```python
from build123d import *

# Parameters (mm, degrees)
SKETCH1_R           = 17.5
BOSS_EXTRUDE1_DEPTH = 15
BOSS_EXTRUDE2_DEPTH = 2
CUT_EXTRUDE1_REACH  = 19
SKETCH3_R           = 3.25
SKETCH4_R           = 1
CUT_EXTRUDE2_DEPTH  = 5
CIRPATTERN1_COUNT   = 4
SKETCH5_R           = 1
CUT_EXTRUDE3_DEPTH  = 2
CIRPATTERN2_COUNT   = 4
SKETCH6_R           = 7.5
CUT_EXTRUDE4_DEPTH  = 5
CUT_EXTRUDE6_START  = -4
SKETCH7_R           = 17.5
SKETCH7_R_2         = 12.5
CUT_EXTRUDE6_DEPTH  = 0.2
FILLET1_R           = 2
CUT_EXTRUDE7_DEPTH  = 3
SKETCH9_R           = 17.5
SKETCH9_R_2         = 16.5
BOSS_EXTRUDE3_DEPTH = 10
SKETCH10_R          = 16.5
BOSS_EXTRUDE4_DEPTH = 1
CUT_EXTRUDE8_DEPTH  = 5
SKETCH12_R          = 1
CUT_EXTRUDE9_DEPTH  = 1
CIRPATTERN3_COUNT   = 4


with BuildPart() as part:
    # Sketch1 → Boss-Extrude1 (new body)
    with BuildSketch(Plane(origin=(0, 0, 0), x_dir=(1, 0, 0), z_dir=(0, 1, 0))):
        Circle(SKETCH1_R)
    extrude(amount=BOSS_EXTRUDE1_DEPTH)

    # Sketch2 → Boss-Extrude2 (add)
    with BuildSketch(Plane(origin=(0, 15, 0), x_dir=(1, 0, 0), z_dir=(0, 1, 0))):
        Polygon((7.3, 0), (3.65, 6.321985448), (-3.65, 6.321985448), (-7.3, 0), (-3.65, -6.321985448), (3.65, -6.321985448), align=None)
    extrude(amount=BOSS_EXTRUDE2_DEPTH)

    # Sketch3 → Cut-Extrude1 (cut, up to next)
    with BuildSketch(Plane.XZ, mode=Mode.PRIVATE) as cut_extrude1_sk1:
        Circle(SKETCH3_R)
    cut_extrude1_tool1 = extrude(cut_extrude1_sk1.sketch, amount=-CUT_EXTRUDE1_REACH, mode=Mode.PRIVATE) & part.part
    add(cut_extrude1_tool1.solids().sort_by_distance((0, 0, 0))[0], mode=Mode.SUBTRACT)

    # Sketch4 → Cut-Extrude2 (cut)
    with BuildSketch(Plane.XZ):
        with Locations((0, 9.5)):
            Circle(SKETCH4_R)
    cut_extrude2 = extrude(amount=-CUT_EXTRUDE2_DEPTH, mode=Mode.SUBTRACT)

    # CirPattern1: Cut-Extrude2 ×4 about axis
    cirpattern1_axis = Axis((0, 0, 0), (0, 1, 0))
    for i in range(1, CIRPATTERN1_COUNT):
        add(cut_extrude2.rotate(cirpattern1_axis, i * 360 / CIRPATTERN1_COUNT), mode=Mode.SUBTRACT)

    # Sketch5 → Cut-Extrude3 (cut)
    with BuildSketch(Plane(origin=(0, 15, 0), x_dir=(1, 0, 0), z_dir=(0, 1, 0))):
        with Locations((0, 14.5)):
            Circle(SKETCH5_R)
    cut_extrude3 = extrude(amount=-CUT_EXTRUDE3_DEPTH, mode=Mode.SUBTRACT)

    # CirPattern2: Cut-Extrude3 ×4 about axis
    cirpattern2_axis = Axis((0, 0, 0), (0, 1, 0))
    for i in range(1, CIRPATTERN2_COUNT):
        add(cut_extrude3.rotate(cirpattern2_axis, i * 360 / CIRPATTERN2_COUNT), mode=Mode.SUBTRACT)

    # Sketch6 → Cut-Extrude4 (cut)
    with BuildSketch(Plane(origin=(0, 15, 0), x_dir=(1, 0, 0), z_dir=(0, 1, 0))):
        Circle(SKETCH6_R)
        Polygon((7.3, 0), (3.65, 6.321985448), (-3.65, 6.321985448), (-7.3, 0), (-3.65, -6.321985448), (3.65, -6.321985448), align=None, mode=Mode.SUBTRACT)
    extrude(amount=-CUT_EXTRUDE4_DEPTH, mode=Mode.SUBTRACT)

    # Sketch7 → Cut-Extrude6 (cut)
    with BuildSketch(Plane(origin=(0, 15, 0), x_dir=(1, 0, 0), z_dir=(0, 1, 0)).offset(CUT_EXTRUDE6_START)):
        Circle(SKETCH7_R)
        Circle(SKETCH7_R_2, mode=Mode.SUBTRACT)
    extrude(amount=-CUT_EXTRUDE6_DEPTH, mode=Mode.SUBTRACT)

    # Fillet1
    fillet1_edges = [part.edges().sort_by_distance(p)[0] for p in [
        (-7.3, 13.5, 0),
        (-3.65, 13.5, 6.321985448),
        (3.65, 13.5, 6.321985448),
        (7.3, 13.5, 0),
        (3.65, 13.5, -6.321985448),
        (-3.65, 13.5, -6.321985448),
    ]]
    fillet(fillet1_edges, radius=FILLET1_R)

    # Sketch8 → Cut-Extrude7 (cut)
    with BuildSketch(Plane(origin=(0, 15, 0), x_dir=(1, 0, 0), z_dir=(0, 1, 0))):
        with BuildLine():
            Line((8.042991645, 14.406952676), (5.21456452, 11.578525551))
            Line((5.21456452, 11.578525551), (11.578525551, 5.21456452))
            Line((11.578525551, 5.21456452), (14.406952676, 8.042991645))
            ThreePointArc((14.406952676, 8.042991645), (11.66726189, 11.66726189), (8.042991645, 14.406952676))
        make_face()
    extrude(amount=-CUT_EXTRUDE7_DEPTH, mode=Mode.SUBTRACT)

    # Sketch9 → Boss-Extrude3 (add)
    with BuildSketch(Plane(origin=(0, 15, 0), x_dir=(1, 0, 0), z_dir=(0, 1, 0))):
        Circle(SKETCH9_R)
        Circle(SKETCH9_R_2, mode=Mode.SUBTRACT)
    extrude(amount=BOSS_EXTRUDE3_DEPTH)

    # Sketch10 → Boss-Extrude4 (add)
    with BuildSketch(Plane(origin=(0, 25, 0), x_dir=(1, 0, 0), z_dir=(0, 1, 0))):
        Circle(SKETCH10_R)
    extrude(amount=-BOSS_EXTRUDE4_DEPTH)

    # Sketch11 → Cut-Extrude8 (cut)
    with BuildSketch(Plane(origin=(0, 25, 0), x_dir=(1, 0, 0), z_dir=(0, 1, 0))):
        with BuildLine():
            Line((5.21456452, 11.578525551), (11.578525551, 5.21456452))
            Line((11.578525551, 5.21456452), (15.140241258, 8.776280228))
            ThreePointArc((15.140241258, 8.776280228), (12.374368671, 12.374368671), (8.776280228, 15.140241258))
            Line((8.776280228, 15.140241258), (5.21456452, 11.578525551))
        make_face()
    extrude(amount=-CUT_EXTRUDE8_DEPTH, mode=Mode.SUBTRACT)

    # Sketch12 → Cut-Extrude9 (cut)
    with BuildSketch(Plane(origin=(0, 25, 0), x_dir=(1, 0, 0), z_dir=(0, 1, 0))):
        with Locations((0, 10)):
            Circle(SKETCH12_R)
    cut_extrude9 = extrude(amount=-CUT_EXTRUDE9_DEPTH, mode=Mode.SUBTRACT)

    # CirPattern3: Cut-Extrude9 ×4 about axis
    cirpattern3_axis = Axis((0, 0, 0), (0, 1, 0))
    for i in range(1, CIRPATTERN3_COUNT):
        add(cut_extrude9.rotate(cirpattern3_axis, i * 360 / CIRPATTERN3_COUNT), mode=Mode.SUBTRACT)


solid = part.part
```
Could you check a few things on this model? Use its own coordinates, in mm. A direction names the side the tool comes from. Coordinates: 2 decimals unless noted, no trailing zeros. Loops run counter-clockwise (first coordinate to the right, second up) from the corner with the lowest first, then second, coordinate; pieces in that order, holes last. Notation, with made-up numbers: M 48.25,42.5 L 70.25,42.5 A17 cw 70.25,74.5 Z; hole C -34,8 d11. An arc over 180 degrees is marked long. Put each result on its own line as item: value. Start each with the question number.
(1) Suppose I cut it at B-B on y = 16. Please give me the cut outline in (x, z).
(2) I need wall thicknesses on line 1 (X direction, y = 24.75, z = 0); line 2 (Y direction, x = -8, z = -10); line 3 (Z direction, x = 0, y = 14.2). Which ranges of each line are inside material? Lowest first, please. Write a range as from..to.
(3) Suppose I cut it at D-D on z = 8. Please give me the cut outline in (x, y), then the cut area to 3 significant figures.
(4) Suppose I cut it at A-A on y = 13.5. Count the separate pieces of the cut face and the enclosed holes in it, then the cut area to 3 significant figures.
(5) Suppose I cut it at C-C on x = -14.5. Please give me the cut outline in (y, z), then the cut area to 3 significant figures.
(6) Will these pins go through, and if not, where does the flat tip stop? P1, Ø1.5, axis at y = 21, z = -12, coming from the +X side; P2, Ø1, axis at y = 5, z = -11, coming from the +X side; P3, Ø3, axis at y = 15, z = 6, coming from the +X side.
(7) Thinking about a two-plate mould opening in X: for faces 1 (the face through (-0.217, 14.014, -13.524)), 2 (the face through (0, 5, 10)), 3 (the face through (-3.794, 17.902, 17.084)), 4 (the face through (8, 11, 11)), which applies, pulls with the +X half, pulls with the -X half, needs draft (parallel to the pull), parting line crosses it, or undercut?
(8) For faces 5 (the face through (-10, 5, 0)), 6 (the face through (-5.46, 13.45, -3.19)), which set-ups out of +Z, -Z, +X, -X, +Y, -Y let a thin tool reach every point of the face, with its end or its side?
Solutions:
1. outline: C 0,0 d35; M -6.72,-1 L -4.23,-5.32 A2 ccw -2.5,-6.32 L 2.5,-6.32 A2 ccw 4.23,-5.32 L 6.72,-1 A2 ccw 6.72,1 L 4.23,5.32 A2 ccw 2.5,6.32 L -2.5,6.32 A2 ccw -4.23,5.32 L -6.72,1 A2 ccw Z; hole C 0,0 d33; hole C 0,0 d6.5
2. line 1: x = -17.5..-11, -9..9, 11..17.5
2. line 2: y = 0..10.8, 11..15, 24..25
2. line 3: z = -17.5..-15.5, -13.5..-7.5, -6.32..-3.25, 3.25..6.32, 7.5..13.5, 15.5..17.5
3. outline: M -15.56,0 L 15.56,0 L 15.56,10.8 L 9.6,10.8 L 9.6,11 L 15.56,11 L 15.56,25 L -15.56,25 L -15.56,11 L -9.6,11 L -9.6,10.8 L -15.56,10.8 Z; hole M -14.43,15 L 14.43,15 L 14.43,24 L -14.43,24 Z
3. area: 516 mm2
4. separate pieces: 2
4. enclosed holes: 7
4. area: 837 mm2
5. outline: M 0,-9.8 L 10.8,-9.8 L 10.8,9.8 L 0,9.8 Z; M 11,-9.8 L 25,-9.8 L 25,9.8 L 11,9.8 Z; hole M 13,-1 L 15,-1 L 15,-7.87 L 24,-7.87 L 24,7.87 L 15,7.87 L 15,1 L 13,1 Z
5. area: 340 mm2
6. P1: stops at x = -10.47
6. P2: stops at x = 14
6. P3: stops at x = 16.91
7. face 1: undercut
7. face 2: undercut
7. face 3: parting line crosses it
7. face 4: needs draft
8. face 5: -Y
8. face 6: none
